Autodesk Inventor part; units mm, degrees
ref_plane "YZ Plane" through (0, 0, 0) normal (1, 0, 0) x (0, 1, 0)
ref_plane "XZ Plane" through (0, 0, 0) normal (0, 1, 0) x (-1, 0, 0)
ref_plane "XY Plane" through (0, 0, 0) normal (0, 0, 1) x (1, 0, 0)
sketch "Sketch1" plane through (0, 0, 0) normal (0, 0, 1) x (1, 0, 0)
  line L0 (-50, 75) -> (50, 75)
  line L1 (50, 75) -> (50, -75)
  line L2 (50, -75) -> (-50, -75)
  line L3 (-50, -75) -> (-50, 75)
  point P0 (0, 0)
  point P1 (0, 75)
  point P2 (-50, 0)
  dimension "d0" = 100
  dimension "d1" = 150
extrude "Extrusion1" add sketch "Sketch1" along normal blind 25
sketch "Sketch2" plane through (0, 0, 0) normal (0, 0, -1) x (-1, 0, 0)
  line L0 (50, -75) -> (-50, -75)
  line L1 (-50, 75) -> (50, 75)
  line L2 (-50, -75) -> (50, 75) construction
  circle A0 centre (0, 0) radius 8
  line L3 (0, 0) -> (-25, 0) construction
  circle A1 centre (-25, 0) radius 8
  dimension "d4" = 16
  dimension "d5" = 25
  dimension "d6" = 16
extrude "Extrusion2" cut sketch "Sketch2" against normal through all
pattern_circular "Circular Pattern1" count 8 over 360 about axis through (0, 0, 0) along (0, 0, 1) of "Extrusion2"
properties part number "Foam_Top_Big_Mic" material "Polystyrene, Expanded"
Input: part model. Units: mm. Frame: model coordinates. Give positions to 0.01 mm unless a question says otherwise; leave off trailing zeros. Loops run counter-clockwise (first coordinate to the right, second up) from the corner with the lowest first, then second, coordinate; pieces in that order, holes last. Notation, with made-up numbers: M -19.5,55.25 L 15.5,55.25 A25 ccw 15.5,67.25 Z; hole C 49.25,-16.5 d8. An arc over 180 degrees is marked long. Answer as CSV lines item,"result". Start each with the question number.
1. Section D-D on z = 16. State how many separate pieces and enclosed holes the cut face has, plus the area to 3 significant figures.
2. Pull-direction query (X, two-part tool) for faces 1 (the face through (50, 1, 12)), 2 (the face through (1, -75, 12)), 3 (the face through (-13.981, 10.583, 12.325)); classes: released by +X, released by -X, zero draft, split by the parting line, or undercut.
3. Section A-A on x = 0. Return loops of the section in (y, z), plus the area to 3 significant figures.
4. Section C-C on y = -28.5. Return loops of the section in (x, z), plus the area to 3 significant figures.
5. Line query: L1, parallel to X at y = -11.5, z = 2.75; L2, parallel to Y at x = 22.5, z = 4.5; L3, parallel to X at y = 18, z = 8. Output: solid intervals per line, ascending.
6. Section B-B on y = 0. Return loops of the section in (x, z).
Computed values:
1,separate pieces,"1"
1,enclosed holes,"9"
1,area,"13,200 mm²"
2,face 1,"released by +X"
2,face 2,"zero draft"
2,face 3,"undercut"
3,outline,"M -75,0 L -33,0 L -33,25 L -75,25 Z; M -17,0 L -8,0 L -8,25 L -17,25 Z; M 8,0 L 17,0 L 17,25 L 8,25 Z; M 33,0 L 75,0 L 75,25 L 33,25 Z"
3,area,"2,550 mm²"
4,outline,"M -50,0 L -7.19,0 L -7.19,25 L -50,25 Z; M 7.19,0 L 50,0 L 50,25 L 7.19,25 Z"
4,area,"2,140 mm²"
5,L1,"x = -50 to -22.76, -12.59 to 12.59, 22.76 to 50"
5,L2,"y = -75 to -24.06, -11.29 to -7.6, 7.6 to 11.29, 24.06 to 75"
5,L3,"x = -50 to -25.67, -9.68 to -3.87, 3.87 to 9.68, 25.67 to 50"
6,outline,"M -50,0 L -33,0 L -33,25 L -50,25 Z; M -17,0 L -8,0 L -8,25 L -17,25 Z; M 8,0 L 17,0 L 17,25 L 8,25 Z; M 33,0 L 50,0 L 50,25 L 33,25 Z"
